```python
from build123d import *

# Parameters (mm, degrees)
SKETCH1_R               = 101.6
BOSS_EXTRUDE1_DEPTH     = 76.2
CUT_EXTRUDE7_DEPTH      = 163.639355631
CUT_EXTRUDE7_DEPTH_BACK = 163.639355631
SKETCH3_R               = 25.4
BOSS_EXTRUDE2_DEPTH     = 76.2


with BuildPart() as part:
    # Sketch1 → Boss-Extrude1 (new body)
    with BuildSketch(Plane.XY):
        with Locations(Location((0, 0, 0), (0, 0, 180))):
            Circle(SKETCH1_R)
    extrude(amount=BOSS_EXTRUDE1_DEPTH)

    # Sketch2 → Cut-Extrude7 (cut, two sides: drawn at the far end of the back side and taken through both)
    with BuildSketch(Plane.XY.offset(76.2).offset(-CUT_EXTRUDE7_DEPTH_BACK)):
        with BuildLine():
            ThreePointArc((-55.703026842, -24.462175809), (-80.165202651, 0), (-55.703026842, 24.462175809))
            Line((-55.703026842, 24.462175809), (-55.703026842, -24.462175809))
        make_face()
        with BuildLine():
            Line((55.703026842, 24.462175809), (55.703026842, -24.462175809))
            ThreePointArc((55.703026842, -24.462175809), (80.165202651, 0), (55.703026842, 24.462175809))
        make_face()
    extrude(amount=CUT_EXTRUDE7_DEPTH + CUT_EXTRUDE7_DEPTH_BACK, mode=Mode.SUBTRACT)

    # Sketch3 → Boss-Extrude2 (add)
    with BuildSketch(Plane.XY.offset(76.2)):
        with Locations(Location((0, 0, 0), (0, 0, 180))):
            Circle(SKETCH3_R)
    extrude(amount=BOSS_EXTRUDE2_DEPTH)


solid = part.part
```
Geometry: final body of the model. Coordinates: model frame, mm. A direction names the side the tool comes from. Round coordinates to 2 decimals unless told otherwise and drop trailing zeros. Write each loop counter-clockwise with the first axis right and the second up, starting at its lowest first coordinate (ties: lowest second). Pieces come first, ordered by that corner, then holes. Notation, with made-up numbers: (65, -28) -> (118, -28) arc R26 ccw to (118, -7) -> close; hole circle Ø5 at (4, 79.25). An arc over 180 degrees is marked (long way). Use CSV: the item, a comma, the result in double quotes. Start each with the question number.
Q1. Section A-A (y = 0). Return loops of the section in (x, z), plus the area to 3 significant figures.
Q2. Section C-C (x = 0). Return loops of the section in (y, z).
Q3. First-contact query: pin 1 Ø10 at (y, z) = (-53, 29) entering from -X; pin 2 Ø1 at (x, y) = (11.5, -31.5) entering from +Z; pin 3 Ø12 at (x, z) = (-35, 43) entering from +Y. Flat tips, straight axial feed; report the tip coordinate or a pass-through.
Q4. Section B-B (z = 16). Return loops of the section in (x, y), plus the area to 3 significant figures.
Q5. Section D-D (x = -61.5). Return loops of the section in (y, z).
Q6. Line query: L1, parallel to Z at x = -12, y = -23.5; L2, parallel to X at y = 61, z = 27.5; L3, parallel to X at y = 58, z = 59. Output: solid intervals per line, ascending.
Q7. Pull-direction query (X, two-part tool) for faces 4 (the face through (-80.16, -0.54, 37.57)), 5 (the face through (-11.721, 22.534, 113.767)), 6 (the face through (1, -1, 0)); classes: pulls with the +X half, pulls with the -X half, needs draft (parallel to the pull), parting line crosses it, or undercut.
Q8. Reachability of faces 1 (the face through (0, 0, 152.4)), 2 (the face through (-21, 21, 76.2)), 3 (the face through (-55.703, 0, 38)) from +Z, -Z, +X, -X, +Y, -Y: full face, straight path, thin tool, end or side. Return the list, or none.
Result sheet:
1,outline,"(-101.6, 0) -> (-80.17, 0) -> (-80.17, 76.2) -> (-101.6, 76.2) -> close; (-55.7, 0) -> (55.7, 0) -> (55.7, 76.2) -> (25.4, 76.2) -> (25.4, 152.4) -> (-25.4, 152.4) -> (-25.4, 76.2) -> (-55.7, 76.2) -> close; (80.17, 0) -> (101.6, 0) -> (101.6, 76.2) -> (80.17, 76.2) -> close"
1,area,"15,600 mm²"
2,outline,"(-101.6, 0) -> (101.6, 0) -> (101.6, 76.2) -> (25.4, 76.2) -> (25.4, 152.4) -> (-25.4, 152.4) -> (-25.4, 76.2) -> (-101.6, 76.2) -> close"
3,pin 1,"x = -89.55"
3,pin 2,"z = 76.2"
3,pin 3,"y = 97.37"
4,outline,"circle Ø203.2 at (0, 0); hole (-55.7, -24.46) -> (-55.7, 24.46) arc R24.46 ccw to start; hole (55.7, -24.46) arc R24.46 ccw to (55.7, 24.46) -> close"
4,area,"30,500 mm²"
5,outline,"(-80.87, 0) -> (-23.77, 0) -> (-23.77, 76.2) -> (-80.87, 76.2) -> close; (23.77, 0) -> (80.87, 0) -> (80.87, 76.2) -> (23.77, 76.2) -> close"
6,L1,"0 to 76.2"
6,L2,"-81.25 to 81.25"
6,L3,"-83.42 to 83.42"
7,face 4,"undercut"
7,face 5,"parting line crosses it"
7,face 6,"needs draft"
8,face 1,"+Z, +X, -X, +Y, -Y"
8,face 2,"+Z"
8,face 3,"+Z, -Z"
